For this review, take the finished solid that the model builds, in its own axes (mm). A direction names the side the tool comes from. Coordinates: 2 decimals unless noted, no trailing zeros. Order: outer loops, then holes, each group sorted by start corner. A loop starts at its lowest first (then second) coordinate and runs counter-clockwise, first axis right, second up.
from build123d import *

# Parameters (mm, degrees)
F0_W     = 3.5
F0_H     = 1.5
F1_DEPTH = 35
F2_DEPTH = 1.5
F3_SIZE  = 1
F4_DEPTH = 7.3


with BuildPart() as f1:
    # F0 (on Top) → F1 (new body)
    with BuildSketch(Plane.XY):
        with BuildLine():
            ThreePointArc((-9.5, 0.394493346), (-8.2992202699, 1.0560835668), (-7.425, 0))
            Line((-7.425, 0), (-2.75, 0))
            ThreePointArc((-2.75, 0), (-2.314413618, 1.4852574204), (-1.1456439237, 2.5))
            Line((-1.1456439237, 2.5), (-9.5, 2.5))
            Line((-9.5, 2.5), (-9.5, 0.394493346))
        make_face()
        with BuildLine():
            ThreePointArc((-9.5, -0.394493346), (-9.575, 0), (-9.5, 0.394493346))
            Line((-9.5, 0.394493346), (-9.5, 2.5))
            Line((-9.5, 2.5), (-13, 2.5))
            Line((-13, 2.5), (-13, 0))
            Line((-13, 0), (-13, -2.5))
            Line((-13, -2.5), (-9.5, -2.5))
            Line((-9.5, -2.5), (-9.5, -0.394493346))
        make_face()
        with BuildLine():
            Line((-2.75, 0), (-7.425, 0))
            ThreePointArc((-7.425, 0), (-8.2992202699, -1.0560835668), (-9.5, -0.394493346))
            Line((-9.5, -0.394493346), (-9.5, -2.5))
            Line((-9.5, -2.5), (-1.1456439237, -2.5))
            ThreePointArc((-1.1456439237, -2.5), (-2.314413618, -1.4852574204), (-2.75, 0))
        make_face()
        Polygon((-13, -4), (-13, -2.5), (-25.5, 0), (-33, 0), align=None)
        Polygon((-25.5, 0), (-13, 2.5), (-13, 4), (-33, 0), align=None)
        Polygon((13, -2.5), (13, -4), (33, 0), (25.5, 0), align=None)
        Polygon((33, 0), (13, 4), (13, 2.5), (25.5, 0), align=None)
        Polygon((-25.5, 0), (-13, -2.5), (-13, 0), align=None)
        Polygon((-13, 0), (-13, 2.5), (-25.5, 0), align=None)
        with Locations((-11.25, 3.25)):
            Rectangle(F0_W, F0_H)
        with BuildLine():
            Line((-9.5, 4), (-9.5, 2.5))
            Line((-9.5, 2.5), (-1.1456439237, 2.5))
            ThreePointArc((-1.1456439237, 2.5), (0, 2.75), (1.1456439237, 2.5))
            Line((1.1456439237, 2.5), (9.5, 2.5))
            Line((9.5, 2.5), (9.5, 4))
            Line((9.5, 4), (-9.5, 4))
        make_face()
        with Locations((11.25, 3.25)):
            Rectangle(F0_W, F0_H)
        with Locations((11.25, -3.25)):
            Rectangle(F0_W, F0_H)
        with BuildLine():
            Line((-1.1456439237, -2.5), (-9.5, -2.5))
            Line((-9.5, -2.5), (-9.5, -4))
            Line((-9.5, -4), (9.5, -4))
            Line((9.5, -4), (9.5, -2.5))
            Line((9.5, -2.5), (1.1456439237, -2.5))
            ThreePointArc((1.1456439237, -2.5), (0, -2.75), (-1.1456439237, -2.5))
        make_face()
        with Locations((-11.25, -3.25)):
            Rectangle(F0_W, F0_H)
        Polygon((13, 0), (13, -2.5), (25.5, 0), align=None)
        Polygon((25.5, 0), (13, 2.5), (13, 0), align=None)
        with BuildLine():
            Line((9.5, 2.5), (9.5, 0.394493346))
            ThreePointArc((9.5, 0.394493346), (9.5560835668, 0.2007797301), (9.575, 0))
            ThreePointArc((9.575, 0), (9.5560835668, -0.2007797301), (9.5, -0.394493346))
            Line((9.5, -0.394493346), (9.5, -2.5))
            Line((9.5, -2.5), (13, -2.5))
            Line((13, -2.5), (13, 0))
            Line((13, 0), (13, 2.5))
            Line((13, 2.5), (9.5, 2.5))
        make_face()
        with BuildLine():
            ThreePointArc((1.1456439237, 2.5), (2.314413618, 1.4852574204), (2.75, 0))
            Line((2.75, 0), (7.425, 0))
            ThreePointArc((7.425, 0), (8.2992202699, 1.0560835668), (9.5, 0.394493346))
            Line((9.5, 0.394493346), (9.5, 2.5))
            Line((9.5, 2.5), (1.1456439237, 2.5))
        make_face()
        with BuildLine():
            Line((7.425, 0), (2.75, 0))
            ThreePointArc((2.75, 0), (2.314413618, -1.4852574204), (1.1456439237, -2.5))
            Line((1.1456439237, -2.5), (9.5, -2.5))
            Line((9.5, -2.5), (9.5, -0.394493346))
            ThreePointArc((9.5, -0.394493346), (8.2992202699, -1.0560835668), (7.425, 0))
        make_face()
    extrude(amount=F1_DEPTH)

    # F0 (on Top) → F2 (join)
    with BuildSketch(Plane.XY):
        Polygon((-13, -4), (-13, -2.5), (-25.5, 0), (-33, 0), align=None)
        Polygon((-25.5, 0), (-13, 2.5), (-13, 4), (-33, 0), align=None)
        with Locations((-11.25, 3.25)):
            Rectangle(F0_W, F0_H)
        with BuildLine():
            Line((-9.5, 4), (-9.5, 2.5))
            Line((-9.5, 2.5), (-1.1456439237, 2.5))
            ThreePointArc((-1.1456439237, 2.5), (0, 2.75), (1.1456439237, 2.5))
            Line((1.1456439237, 2.5), (9.5, 2.5))
            Line((9.5, 2.5), (9.5, 4))
            Line((9.5, 4), (-9.5, 4))
        make_face()
        with Locations((11.25, 3.25)):
            Rectangle(F0_W, F0_H)
        Polygon((-13, 0), (-13, 2.5), (-25.5, 0), align=None)
        Polygon((-25.5, 0), (-13, -2.5), (-13, 0), align=None)
        with BuildLine():
            ThreePointArc((-9.5, 0.394493346), (-8.2992202699, 1.0560835668), (-7.425, 0))
            Line((-7.425, 0), (-2.75, 0))
            ThreePointArc((-2.75, 0), (-2.314413618, 1.4852574204), (-1.1456439237, 2.5))
            Line((-1.1456439237, 2.5), (-9.5, 2.5))
            Line((-9.5, 2.5), (-9.5, 0.394493346))
        make_face()
        with BuildLine():
            ThreePointArc((-9.5, -0.394493346), (-9.575, 0), (-9.5, 0.394493346))
            Line((-9.5, 0.394493346), (-9.5, 2.5))
            Line((-9.5, 2.5), (-13, 2.5))
            Line((-13, 2.5), (-13, 0))
            Line((-13, 0), (-13, -2.5))
            Line((-13, -2.5), (-9.5, -2.5))
            Line((-9.5, -2.5), (-9.5, -0.394493346))
        make_face()
        with BuildLine():
            Line((-2.75, 0), (-7.425, 0))
            ThreePointArc((-7.425, 0), (-8.2992202699, -1.0560835668), (-9.5, -0.394493346))
            Line((-9.5, -0.394493346), (-9.5, -2.5))
            Line((-9.5, -2.5), (-1.1456439237, -2.5))
            ThreePointArc((-1.1456439237, -2.5), (-2.314413618, -1.4852574204), (-2.75, 0))
        make_face()
        with Locations((11.25, -3.25)):
            Rectangle(F0_W, F0_H)
        with BuildLine():
            Line((-1.1456439237, -2.5), (-9.5, -2.5))
            Line((-9.5, -2.5), (-9.5, -4))
            Line((-9.5, -4), (9.5, -4))
            Line((9.5, -4), (9.5, -2.5))
            Line((9.5, -2.5), (1.1456439237, -2.5))
            ThreePointArc((1.1456439237, -2.5), (0, -2.75), (-1.1456439237, -2.5))
        make_face()
        with Locations((-11.25, -3.25)):
            Rectangle(F0_W, F0_H)
        Polygon((13, -2.5), (13, -4), (33, 0), (25.5, 0), align=None)
        Polygon((13, 0), (13, -2.5), (25.5, 0), align=None)
        Polygon((25.5, 0), (13, 2.5), (13, 0), align=None)
        Polygon((33, 0), (13, 4), (13, 2.5), (25.5, 0), align=None)
        with BuildLine():
            ThreePointArc((1.1456439237, 2.5), (2.314413618, 1.4852574204), (2.75, 0))
            Line((2.75, 0), (7.425, 0))
            ThreePointArc((7.425, 0), (8.2992202699, 1.0560835668), (9.5, 0.394493346))
            Line((9.5, 0.394493346), (9.5, 2.5))
            Line((9.5, 2.5), (1.1456439237, 2.5))
        make_face()
        with BuildLine():
            Line((7.425, 0), (2.75, 0))
            ThreePointArc((2.75, 0), (2.314413618, -1.4852574204), (1.1456439237, -2.5))
            Line((1.1456439237, -2.5), (9.5, -2.5))
            Line((9.5, -2.5), (9.5, -0.394493346))
            ThreePointArc((9.5, -0.394493346), (8.2992202699, -1.0560835668), (7.425, 0))
        make_face()
        with BuildLine():
            Line((9.5, 2.5), (9.5, 0.394493346))
            ThreePointArc((9.5, 0.394493346), (9.5560835668, 0.2007797301), (9.575, 0))
            ThreePointArc((9.575, 0), (9.5560835668, -0.2007797301), (9.5, -0.394493346))
            Line((9.5, -0.394493346), (9.5, -2.5))
            Line((9.5, -2.5), (13, -2.5))
            Line((13, -2.5), (13, 0))
            Line((13, 0), (13, 2.5))
            Line((13, 2.5), (9.5, 2.5))
        make_face()
    extrude(amount=-F2_DEPTH)

    # F3
    f3_edges = [f1.edges().sort_by_distance(p)[0] for p in [
        (-9.575, 0, -1.5),
        (7.5, -0.394493, -1.5),
        (1.145644, -2.5, -1.5),
    ]]
    chamfer(f3_edges, length=F3_SIZE)

    # F0 (on Top) → F4 (join)
    with BuildSketch(Plane.XY):
        with Locations((-11.25, 3.25)):
            Rectangle(F0_W, F0_H)
        with Locations((11.25, 3.25)):
            Rectangle(F0_W, F0_H)
        Polygon((-25.5, 0), (-13, 2.5), (-13, 4), (-33, 0), align=None)
        Polygon((-13, -4), (-13, -2.5), (-25.5, 0), (-33, 0), align=None)
        with Locations((11.25, -3.25)):
            Rectangle(F0_W, F0_H)
        with Locations((-11.25, -3.25)):
            Rectangle(F0_W, F0_H)
        Polygon((33, 0), (13, 4), (13, 2.5), (25.5, 0), align=None)
        Polygon((13, -2.5), (13, -4), (33, 0), (25.5, 0), align=None)
    extrude(amount=-F4_DEPTH)


solid = f1.part
1. Take a section at B-B, the plane z = 6.5. Give the number of separate pieces and of enclosed holes in the cut face, plus the area to 3 significant figures.
Answer below:
separate pieces: 1
enclosed holes: 3
area: 337 mm2
2. Take a section at D-D, the plane x = -27. Give the boundary of the cut face in (y, z), plus the area to 3 significant figures.
Answer below:
outline: (-1.2, -7.3) - (1.2, -7.3) - (1.2, 35) - (-1.2, 35) - close
area: 102 mm2
3. Take a section at C-C, the plane x = 28.5. Give the boundary of the cut face in (y, z).
Answer below:
outline: (-0.9, -7.3) - (0.9, -7.3) - (0.9, 35) - (-0.9, 35) - close
4. Clearance check with flat-ended pins moving along their axes: pin 1 Ø4 at (x, z) = (-18.5, 17.5) entering from +Y; pin 2 Ø10 at (x, z) = (-21, 21.5) entering from +Y; pin 3 Ø2.5 at (x, y) = (-4, 1.5) entering from -Z. State where each tip first meets the part, or that it passes through.
Answer below:
pin 1: stops at y = 3.3
pin 2: stops at y = 3.4
pin 3: stops at z = -1.5
5. Machinability: for faces 4 (the face through (23, 2, 14)), 5 (the face through (-9.5, -3, -4)), 6 (the face through (11, 2.5, -4)), which of the approach directions +Z, -Z, +X, -X, +Y, -Y give a long, thin tool a straight path to every point of the face, cutting with its end or side? Answer none if there is none.
Answer below:
face 4: +Z, -Z, +X, +Y
face 5: -Z, +Y, -Y
face 6: -Z
6. The part is to be moulded in two halves that separate along Y. For faces 1 (the face through (-19.34, 1.23, -4.36)), 2 (the face through (-20.4, 1.2, -7.3)), 3 (the face through (23, -2, 14)), say which applies: +Y half, -Y half, draft (parallel to the pull), parting line (faces both ways), or undercut.
Answer below:
face 1: undercut
face 2: draft
face 3: -Y half
7. To check wall thickness, follow L1, parallel to Y at x = -2.5, z = 4.5; L2, parallel to Z at x = 17, y = 0.75; L3, parallel to Y at x = -18, z = 11. State the ranges of each line that lie inside material, in increasing order.
Answer below:
L1: y = -4 to -1.15, 1.15 to 4
L2: z = -1.5 to 35
L3: y = -3 to 3
8. Take a section at A-A, the plane x = 17. Give the boundary of the cut face in (y, z), plus the area to 3 significant figures.
Answer below:
outline: (-3.2, -7.3) - (-1.7, -7.3) - (-1.7, -1.5) - (1.7, -1.5) - (1.7, -7.3) - (3.2, -7.3) - (3.2, 35) - (-3.2, 35) - close
area: 251 mm2
